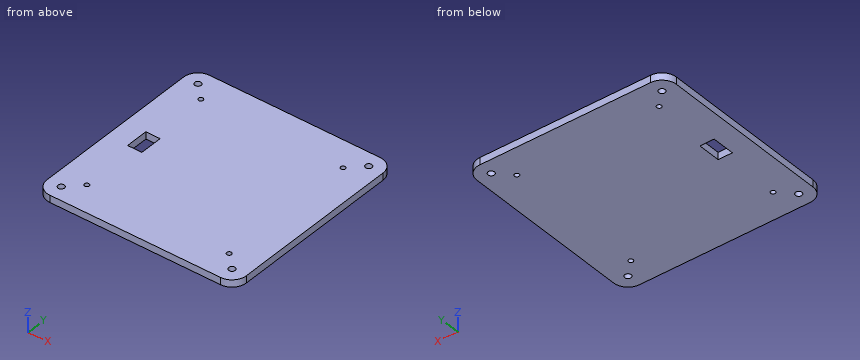
from build123d import *

# Parameters (mm, degrees)
ESKIZ_KONTUR_W        = 10
ESKIZ_KONTUR_H        = 16
PLASTINA_DEPTH        = 5
OTVERSTIYA_DEPTH      = 100.121138008
OTVERSTIYA_DEPTH_BACK = 100.121138008
ESKIZ_OTVERSTIYA_R    = 2.25
ESKIZ_OTVERSTIYA_R_2  = 1.65


with BuildPart() as part:
    # Eskiz_kontur → Plastina (new body)
    with BuildSketch(Plane.XY):
        with BuildLine():
            Line((-70, -60), (-70, 60))
            ThreePointArc((-70, 60), (-67.071067812, 67.071067812), (-60, 70))
            Line((-60, 70), (60, 70))
            ThreePointArc((60, 70), (67.071067812, 67.071067812), (70, 60))
            Line((70, 60), (70, -60))
            ThreePointArc((70, -60), (67.071067812, -67.071067812), (60, -70))
            Line((60, -70), (-60, -70))
            ThreePointArc((-60, -70), (-67.071067812, -67.071067812), (-70, -60))
        make_face()
        with Locations((-50, 0)):
            Rectangle(ESKIZ_KONTUR_W, ESKIZ_KONTUR_H, mode=Mode.SUBTRACT)
    extrude(amount=PLASTINA_DEPTH)

    # Eskiz_otverstiya → Otverstiya (cut, two sides: drawn at the far end of the back side and taken through both)
    with BuildSketch(Plane.XY.offset(-OTVERSTIYA_DEPTH_BACK)):
        with Locations((-60, -60)):
            Circle(ESKIZ_OTVERSTIYA_R)
        with Locations((-50, -50)):
            Circle(ESKIZ_OTVERSTIYA_R_2)
        with Locations((60, -60)):
            Circle(ESKIZ_OTVERSTIYA_R)
        with Locations((50, -50)):
            Circle(ESKIZ_OTVERSTIYA_R_2)
        with Locations((-50, 50)):
            Circle(ESKIZ_OTVERSTIYA_R_2)
        with Locations((-60, 60)):
            Circle(ESKIZ_OTVERSTIYA_R)
        with Locations((50, 50)):
            Circle(ESKIZ_OTVERSTIYA_R_2)
        with Locations((60, 60)):
            Circle(ESKIZ_OTVERSTIYA_R)
    extrude(amount=OTVERSTIYA_DEPTH + OTVERSTIYA_DEPTH_BACK, mode=Mode.SUBTRACT)


solid = part.part
The listing builds one solid part. Answer for the finished solid, in the listing's coordinates (mm). Coordinates: 2 decimals unless noted, no trailing zeros. Order: outer loops, then holes, each group sorted by start corner. A loop starts at its lowest first (then second) coordinate and runs counter-clockwise, first axis right, second up. Notation, with made-up numbers: (71.25, -31) -> (81.25, -31) arc R20 ccw to (81.25, -7) -> close; hole circle Ø3 at (-10.75, 19.5). An arc over 180 degrees is marked (long way). Answer in a Markdown table with one row per item. Add a question column.
Item 1: Each of these flat-tipped pins is pushed along its axis until it touches: P1, Ø4, axis at x = -50, y = 50, coming from the +Z side; P2, Ø2.5, axis at x = 50, y = -50, coming from the -Z side. Where does it stop, or does it pass through?
Item 2: Find the intervals of material crossed by L1, parallel to X at y = 50, z = 3.85; L2, parallel to X at y = 60, z = 1.75, in increasing order. Write a range as from..to.
Item 3: Find section C-C (z = 4.1). State how many separate pieces and enclosed holes the cut face has, then the cut area to 3 significant figures.
Item 4: Find section B-B (x = -50). Write down the section's boundary in (y, z), then the cut area to 3 significant figures.
Item 5: Find section A-A (y = 50). Write down the section's boundary in (x, z).
Result set:
| question | item | result |
|---|---|---|
| 1 | P1 | stops at z = 5 |
| 1 | P2 | passes through |
| 2 | L1 | x = -70..-51.65, -48.35..48.35, 51.65..70 |
| 2 | L2 | x = -70..-62.25, -57.75..57.75, 62.25..70 |
| 3 | separate pieces | 1 |
| 3 | enclosed holes | 9 |
| 3 | area | 19,300 mm² |
| 4 | outline | (-70, 0) -> (-51.65, 0) -> (-51.65, 5) -> (-70, 5) -> close; (-48.35, 0) -> (-8, 0) -> (-8, 5) -> (-48.35, 5) -> close; (8, 0) -> (48.35, 0) -> (48.35, 5) -> (8, 5) -> close; (51.65, 0) -> (70, 0) -> (70, 5) -> (51.65, 5) -> close |
| 4 | area | 587 mm² |
| 5 | outline | (-70, 0) -> (-51.65, 0) -> (-51.65, 5) -> (-70, 5) -> close; (-48.35, 0) -> (48.35, 0) -> (48.35, 5) -> (-48.35, 5) -> close; (51.65, 0) -> (70, 0) -> (70, 5) -> (51.65, 5) -> close |
